from build123d import *

# Parameters (mm, degrees)
F1_DEPTH = 1016
F3_DEPTH = 57.151
F4_W     = 19.05
F4_H     = 38.1
F5_DEPTH = 57.151


# Not quite as in the source:
# - ends of sketch curves that miss each other by under 0.0002 mm in the source are joined


with BuildPart() as f1:
    # F0 (on Top) → F1 (new body)
    with BuildSketch(Plane.XY):
        with BuildLine():
            ThreePointArc((0, 12.7), (3.7197438789, 3.7197438789), (12.7, 0))
            Line((12.7, 0), (15.9004, 0))
            ThreePointArc((15.9004, 0), (18.127503518, 0.922496482), (19.05, 3.1496))
            Line((19.05, 3.1496), (19.05, 34.9504))
            ThreePointArc((19.05, 34.9504), (18.127503518, 37.177503518), (15.9004, 38.1))
            Line((15.9004, 38.1), (3.1496, 38.1))
            ThreePointArc((3.1496, 38.1), (0.922496482, 37.177503518), (0, 34.9504))
            Line((0, 34.9504), (0, 12.7))
        make_face()
        with BuildLine():
            Line((19.05, 34.9504), (19.05, 3.1496))
            ThreePointArc((19.05, 3.1496), (19.972496482, 0.922496482), (22.1996, 0))
            Line((22.1996, 0), (34.9504, 0))
            ThreePointArc((34.9504, 0), (37.177503518, 0.922496482), (38.1, 3.1496))
            Line((38.1, 3.1496), (38.1, 34.9504))
            ThreePointArc((38.1, 34.9504), (37.177503518, 37.177503518), (34.9504, 38.1))
            Line((34.9504, 38.1), (22.1996, 38.1))
            ThreePointArc((22.1996, 38.1), (19.972496482, 37.177503518), (19.05, 34.9504))
        make_face()
        with BuildLine():
            Line((38.1, 34.9504), (38.1, 3.1496))
            ThreePointArc((38.1, 3.1496), (39.022496482, 0.922496482), (41.2496, 0))
            Line((41.2496, 0), (44.45, 0))
            ThreePointArc((44.45, 0), (53.4302561211, 3.7197438789), (57.15, 12.7))
            Line((57.15, 12.7), (57.15, 34.9504))
            ThreePointArc((57.15, 34.9504), (56.227503518, 37.177503518), (54.0004, 38.1))
            Line((54.0004, 38.1), (41.2496, 38.1))
            ThreePointArc((41.2496, 38.1), (39.022496482, 37.177503518), (38.1, 34.9504))
        make_face()
        with BuildLine():
            ThreePointArc((19.0499988437, 41.2496), (19.9724953256, 39.022496482), (22.1995988437, 38.1))
            Line((22.1995988437, 38.1), (34.9504, 38.1))
            Line((34.9504, 38.1), (41.2496, 38.1))
            Line((41.2496, 38.1), (54.0004, 38.1))
            ThreePointArc((54.0004, 38.1), (56.2275023617, 39.022496482), (57.1499988437, 41.2496))
            Line((57.1499988437, 41.2496), (57.1499988437, 44.45))
            ThreePointArc((57.1499988437, 44.45), (53.4302549647, 53.4302561211), (44.4499988437, 57.15))
            Line((44.4499988437, 57.15), (22.1995988437, 57.15))
            ThreePointArc((22.1995988437, 57.15), (19.9724953256, 56.227503518), (19.0499988437, 54.0004))
            Line((19.0499988437, 54.0004), (19.0499988437, 41.2496))
        make_face()
    extrude(amount=F1_DEPTH)

    # F2 (on face) → F3 (cut, through all)
    with BuildSketch(Plane.YZ.offset(57.15)):
        Polygon((57.15, 0), (57.15, 57.15), (0, 0), (12.7, 0), align=None)
        Polygon((12.7, 1016), (0, 1016), (57.15, 958.85), (57.15, 1016), align=None)
    extrude(amount=-F3_DEPTH, mode=Mode.SUBTRACT)

    # F4 (on face) → F5 (cut, through all)
    with BuildSketch(Plane.YZ.offset(57.15)):
        with Locations((9.525, 527.05)):
            Rectangle(F4_W, F4_H)
    extrude(amount=-F5_DEPTH, mode=Mode.SUBTRACT)


solid = f1.part
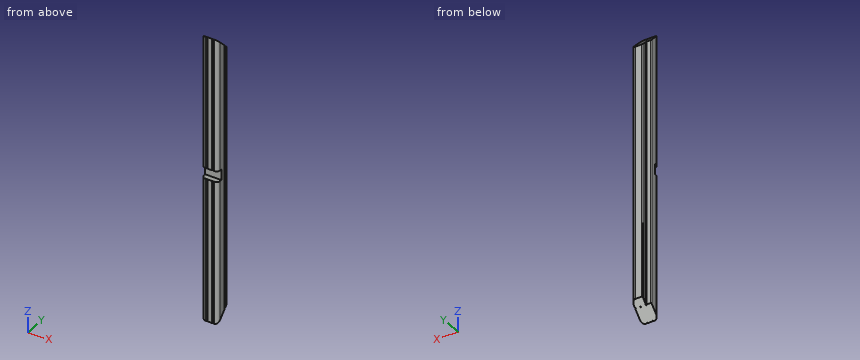
Could you check a few things on this model? Use its own coordinates, in mm. Give positions to 0.01 mm unless a question says otherwise; leave off trailing zeros. Order: outer loops, then holes, each group sorted by start corner. A loop starts at its lowest first (then second) coordinate and runs counter-clockwise, first axis right, second up.
1. Suppose I cut it at A-A (z = 572). List the corners of the cut face in (x, y) for me, plus the area to 3 significant figures.
2. Will these pins go through, and if not, where does the flat tip stop? P1, Ø1.9, axis at x = 38, z = 659.5, coming from the -Y side; P2, Ø1.5, axis at x = 28.5, y = 15, coming from the +Z side; P3, Ø5, axis at x = 32.5, y = 35, coming from the -Z side.
3. I need wall thicknesses on L1, parallel to X at y = 37, z = 499.5; L2, parallel to X at y = 2, z = 353; L3, parallel to Z at x = 41.5, y = 54. Which ranges of each line are inside material? Lowest first, please.
Solved:
1. outline: (0, 12.7) arc R12.7 ccw to (12.7, 0) - (15.9, 0) arc R3.15 ccw to (19.05, 3.15) arc R3.15 ccw to (22.2, 0) - (34.95, 0) arc R3.15 ccw to (38.1, 3.15) arc R3.15 ccw to (41.25, 0) - (44.45, 0) arc R12.7 ccw to (57.15, 12.7) - (57.15, 34.95) arc R3.15 ccw to (54, 38.1) arc R3.15 ccw to (57.15, 41.25) - (57.15, 44.45) arc R12.7 ccw to (44.45, 57.15) - (22.2, 57.15) arc R3.15 ccw to (19.05, 54) - (19.05, 41.25) arc R3.15 ccw to (22.2, 38.1) arc R3.15 ccw to (19.05, 34.95) arc R3.15 ccw to (15.9, 38.1) - (3.15, 38.1) arc R3.15 ccw to (0, 34.95) - close; hole (34.95, 38.1) arc R3.15 cw to (38.1, 34.95) arc R3.15 cw to (41.25, 38.1) - close
1. area: 2,770 mm2
2. P1: stops at y = 0.8
2. P2: stops at z = 1001.75
2. P3: stops at z = 32.5
3. L1: x = 0.76 to 18.29, 19.81 to 37.34, 38.86 to 56.39
3. L2: x = 5.86 to 18.83, 19.27 to 37.88, 38.32 to 51.29
3. L3: z = 54 to 962
